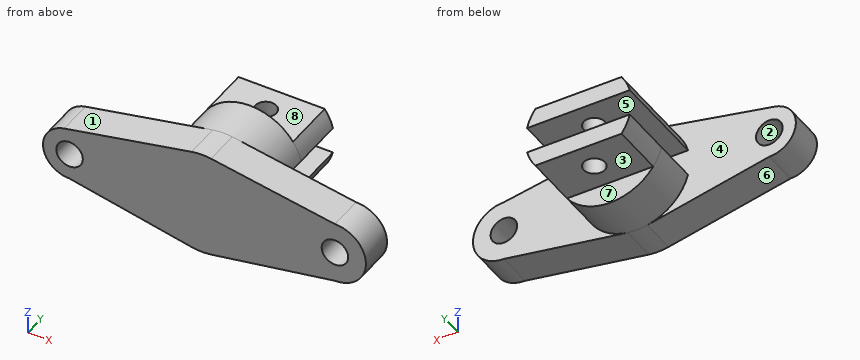
from build123d import *

# Parameters (mm, degrees)
SALIENTE_EXTRUIR1_OUTLINE_R = 7.5
SALIENTE_EXTRUIR1_DEPTH     = 20
SALIENTE_EXTRUIR2_START     = 20
CROQUIS2_4_R                = 7.5
SALIENTE_EXTRUIR2_DEPTH     = 25
SALIENTE_EXTRUIR3_START     = 45
SALIENTE_EXTRUIR3_DEPTH     = 30
CORTAR_EXTRUIR1_DEPTH       = 123.805740908
CORTAR_EXTRUIR1_DEPTH_BACK  = 123.805740908
CROQUIS3_R                  = 6


# Read off the part's stored shape, not the designer's step: Saliente-Extruir1
with BuildPart() as part:
    # Saliente-Extruir1 outline → Saliente-Extruir1 (new body)
    with BuildSketch(Plane(origin=(0, 0, 0), x_dir=(1, 0, 0), z_dir=(0, 1, 0))):
        with BuildLine():
            Line((75, 17.5), (4.980303505, 29.583721487))
            ThreePointArc((4.980303505, 29.583721487), (-0.583157592, 29.994331585), (-6.126453941, 29.367781021))
            Line((-6.126453941, 29.367781021), (-75, 15))
            ThreePointArc((-75, 15), (-89.924042295, 1.50763443), (-78, -14.696938457))
            Line((-78, -14.696938457), (-6, -29.393876913))
            ThreePointArc((-6, -29.393876913), (-0.518609175, -29.995517074), (4.980303505, -29.583721487))
            Line((4.980303505, -29.583721487), (75, -17.5))
            ThreePointArc((75, -17.5), (92.5, 0), (75, 17.5))
        make_face()
        with Locations((-75, 0)):
            Circle(SALIENTE_EXTRUIR1_OUTLINE_R, mode=Mode.SUBTRACT)
        with Locations((75, 0)):
            Circle(SALIENTE_EXTRUIR1_OUTLINE_R, mode=Mode.SUBTRACT)
    extrude(amount=SALIENTE_EXTRUIR1_DEPTH)

    # Croquis2<4> → Saliente-Extruir2 (add)
    with BuildSketch(Plane(origin=(0, 0, 0), x_dir=(1, 0, 0), z_dir=(0, 1, 0)).offset(SALIENTE_EXTRUIR2_START)):
        with Locations(Location((-75, 0, 0), (0, 0, 270))):
            Circle(CROQUIS2_4_R)
        with Locations(Location((75, 0, 0), (0, 0, 270))):
            Circle(CROQUIS2_4_R)
        with BuildLine():
            Line((29.047375097, 7.5), (-29.047375097, 7.5))
            ThreePointArc((-29.047375097, 7.5), (0, 30), (29.047375097, 7.5))
        make_face()
        with BuildLine():
            Line((-29.047375097, -7.5), (29.047375097, -7.5))
            ThreePointArc((29.047375097, -7.5), (0, -30), (-29.047375097, -7.5))
        make_face()
    extrude(amount=SALIENTE_EXTRUIR2_DEPTH)


with BuildPart() as saliente_extruir2_kept_piece:
    # of the separate pieces the step leaves, the one the design keeps (saliente_extruir2_pieces_kept)
    add(part.part.solids().sort_by_distance((4.980303505, 0, 29.583721487))[0])

    # Croquis2<5> → Saliente-Extruir3 (add)
    with BuildSketch(Plane(origin=(0, 0, 0), x_dir=(1, 0, 0), z_dir=(0, 1, 0)).offset(SALIENTE_EXTRUIR3_START)):
        with BuildLine():
            Line((24.366985862, 17.5), (-24.366985862, 17.5))
            ThreePointArc((-24.366985862, 17.5), (-27.171188586, 12.717173855), (-29.047375097, 7.5))
            Line((-29.047375097, 7.5), (29.047375097, 7.5))
            ThreePointArc((29.047375097, 7.5), (27.171188586, 12.717173855), (24.366985862, 17.5))
        make_face()
        with BuildLine():
            ThreePointArc((-29.047375097, -7.5), (-27.171188586, -12.717173855), (-24.366985862, -17.5))
            Line((-24.366985862, -17.5), (24.366985862, -17.5))
            ThreePointArc((24.366985862, -17.5), (27.171188586, -12.717173855), (29.047375097, -7.5))
            Line((29.047375097, -7.5), (-29.047375097, -7.5))
        make_face()
    extrude(amount=SALIENTE_EXTRUIR3_DEPTH)

    # Croquis3 → Cortar-Extruir1 (cut, two sides: drawn at the far end of the back side and taken through both)
    with BuildSketch(Plane.XY.offset(-CORTAR_EXTRUIR1_DEPTH_BACK)):
        with Locations((0, 60)):
            Circle(CROQUIS3_R)
    extrude(amount=CORTAR_EXTRUIR1_DEPTH + CORTAR_EXTRUIR1_DEPTH_BACK, mode=Mode.SUBTRACT)


solid = saliente_extruir2_kept_piece.part
Part model, mm, in its own coordinate system. Face numbers are marked on the shaded views. A direction names the side the tool comes from. Round coordinates to 2 decimals unless told otherwise and drop trailing zeros. Write each loop counter-clockwise with the first axis right and the second up, starting at its lowest first coordinate (ties: lowest second). Pieces come first, ordered by that corner, then holes. Notation, with made-up numbers: M 86,8 L 108,8 A18 ccw 108,17 Z; hole C 53,42 d7. An arc over 180 degrees is marked long. Return JSON: item names as keys, results as strings. Group by question number.
(1) Saw through at B-B on z = 0. Write the cut outline in (x, y), then the cut area to 3 significant figures.
(2) Two-plate mould, pull along X, no slides. Class the marked faces 1, 2 and 3: +X half, -X half, draft (parallel to the pull), parting line (faces both ways), or undercut.
(3) Drill centre lines: probe 1 along X at (y, z) = (13, 0); probe 2 along Z at (x, y) = (-22, 63); probe 3 along Y at (x, z) = (0, -10.5). Where is each one in solid material? Low to high.
(4) Pin check, flat tips, straight feed: pin 1 Ø13.5 at (x, z) = (-10.5, 26) entering from +Y; pin 2 Ø19.5 at (x, z) = (-75, 0) entering from +Y; pin 3 Ø12 at (y, z) = (40, 7.5) entering from -X. Stop position of each tip, or through.
(5) Saw through at D-D on x = 77. Write the cut outline in (y, z), then the cut area to 3 significant figures.
(6) Saw through at A-A on x = 0. Write the cut outline in (y, z), then the cut area to 4 significant figures.
(7) Saw through at C-C on y = 10.5. Write the cut outline in (x, z), then the cut area to 3 significant figures.
(8) Which spindle directions (+Z, -Z, +X, -X, +Y, -Y) get a long thin tool onto all of the face, cutting with end or side? Do the marked faces 4, 5, 6, 7 and 8. Say none if no direction does.
Returned:
{
 "1": {"outline": "M -90,0 L -82.5,0 L -82.5,20 L -90,20 Z; M -67.5,0 L 67.5,0 L 67.5,20 L -67.5,20 Z; M 82.5,0 L 92.5,0 L 92.5,20 L 82.5,20 Z", "area": "3,050 mm²"},
 "2": {"face 1": "-X half", "face 2": "undercut", "face 3": "draft"},
 "3": {"probe 1": "-90 to -82.5, -67.5 to 67.5, 82.5 to 92.5", "probe 2": "-17.5 to -7.5, 7.5 to 17.5", "probe 3": "0 to 54, 66 to 75"},
 "4": {"pin 1": "y = 45", "pin 2": "y = 20", "pin 3": "x = -29.05"},
 "5": {"outline": "M 0,-17.39 L 20,-17.39 L 20,-7.23 L 0,-7.23 Z; M 0,7.23 L 20,7.23 L 20,17.39 L 0,17.39 Z", "area": "406 mm²"},
 "6": {"outline": "M 0,-30 L 45,-30 L 45,-17.5 L 54,-17.5 L 54,-7.5 L 20,-7.5 L 20,7.5 L 54,7.5 L 54,17.5 L 45,17.5 L 45,30 L 0,30 Z; M 66,-17.5 L 75,-17.5 L 75,-7.5 L 66,-7.5 Z; M 66,7.5 L 75,7.5 L 75,17.5 L 66,17.5 Z", "area": "2,685 mm²"},
 "7": {"outline": "M -78,14.7 A15 ccw -75,-15 L -6.13,-29.37 A30 ccw 4.98,-29.58 L 75,-17.5 A17.5 ccw 75,17.5 L 4.98,29.58 A30 ccw -6,29.39 Z; hole C -75,0 d15; hole C 75,0 d15", "area": "7,510 mm²"},
 "8": {"face 4": "+Y", "face 5": "+X, -X, +Y", "face 6": "-Z, -X, +Y, -Y", "face 7": "-Z, +X, -X, +Y", "face 8": "+Z, +X, -X, +Y"}
}
